Read the model definition and answer for the solid it produces. Units are mm, in the model's axes. Face numbers are marked on the shaded views. A direction names the side the tool comes from. Round coordinates to 2 decimals unless told otherwise and drop trailing zeros. Order: outer loops, then holes, each group sorted by start corner. A loop starts at its lowest first (then second) coordinate and runs counter-clockwise, first axis right, second up. Notation, with made-up numbers: (-30, 66) -> (5, 66) arc R6 cw to (5, 75) -> close; hole circle Ø2 at (-21, 16). An arc over 180 degrees is marked (long way). One line per item, written item: value. Start each with the question number.
1. Section B-B (z = 2.25) is taken. Give the vertices of the cut face in (x, y).
2. The mould has two halves that part along Y. Classify the marked faces 1, 2 and 3: released by +Y, released by -Y, zero draft, split by the parting line, or undercut.
3. Section A-A (x = 7.5) is taken. Give the vertices of the cut face in (y, z), then the cut area to 3 significant figures.
4. Section D-D (x = -3) is taken. Give the vertices of the cut face in (y, z).
5. Flat-ended cylindrical pins translate along their axes: pin 1 Ø10 at (x, z) = (-8, 5.5) entering from -Y; pin 2 Ø0.6 at (y, z) = (-16.5, 2.5) entering from -X. Find the tip coordinate at first contact, or state that the pin passes through.
6. Section C-C (y = -4.25) is taken. Give the vertices of the cut face in (x, z), then the cut area to 3 significant figures.
7. Consider line 1 (Y direction, x = 11, z = 3); line 2 (Y direction, x = -18, z = 4.5); line 3 (X direction, y = -15.5, z = 3.5). Determine where each line is inside the solid, lowest interval first.
8. For the marked faces 4, 5 and 6, determine the directions among +Z, -Z, +X, -X, +Y, -Y from which every point of the face is accessible in a straight line to the end or side of a thin tool.
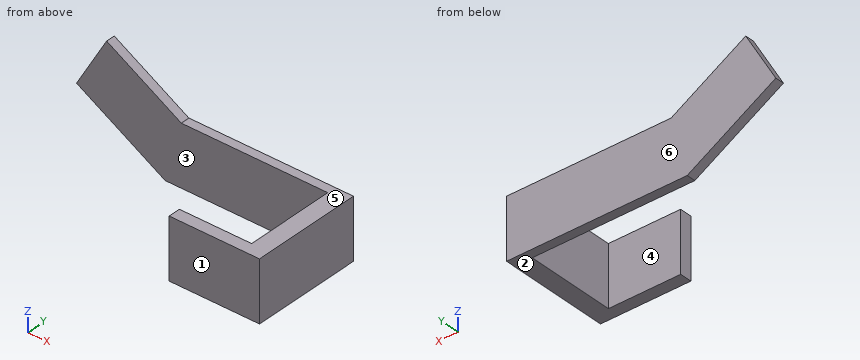
from build123d import *

# Parameters (mm, degrees)
BOSS_EXTRUDE1_DEPTH = 1.5
SKETCH2_W           = 3
SKETCH2_H           = 10
BOSS_EXTRUDE2_DEPTH = 17
SKETCH3_W           = 10
SKETCH3_H           = 2
BOSS_EXTRUDE3_DEPTH = 12


with BuildPart() as part:
    # Sketch1 → Boss-Extrude1 (new body)
    with BuildSketch(Plane(origin=(0, 0, 0), x_dir=(1, 0, 0), z_dir=(0, 1, 0))):
        Polygon((-10.606601718, 3.535533906), (-25.329033582, -4.964466094), (-20.329033582, -13.624720132), (-7.927109793, -6.464466094), (19.393398282, -6.464466094), (19.393398282, 3.535533906), align=None)
    extrude(amount=BOSS_EXTRUDE1_DEPTH)

    # Sketch2 → Boss-Extrude2 (add)
    with BuildSketch(Plane.XZ):
        with Locations((17.893398282, 1.464466094)):
            Rectangle(SKETCH2_W, SKETCH2_H)
    extrude(amount=BOSS_EXTRUDE2_DEPTH)

    # Sketch3 → Boss-Extrude3 (add)
    with BuildSketch(Plane.ZY.offset(-16.393398282)):
        with Locations((1.464466094, -16)):
            Rectangle(SKETCH3_W, SKETCH3_H)
    extrude(amount=BOSS_EXTRUDE3_DEPTH)


solid = part.part
Answer:
1. outline: (-20.63, 0) -> (16.39, 0) -> (16.39, -15) -> (4.39, -15) -> (4.39, -17) -> (19.39, -17) -> (19.39, 1.5) -> (-20.63, 1.5) -> close
2. face 1: released by -Y
2. face 2: zero draft
2. face 3: undercut
3. outline: (-17, -3.54) -> (-15, -3.54) -> (-15, 6.46) -> (-17, 6.46) -> close; (0, -3.54) -> (1.5, -3.54) -> (1.5, 6.46) -> (0, 6.46) -> close
3. area: 35.0 mm^2
4. outline: (0, -3.54) -> (1.5, -3.54) -> (1.5, 6.46) -> (0, 6.46) -> close
5. pin 1: y = 0
5. pin 2: x = 4.39
6. outline: (16.39, -3.54) -> (19.39, -3.54) -> (19.39, 6.46) -> (16.39, 6.46) -> close
6. area: 30.0 mm^2
7. line 1: -17 to -15, 0 to 1.5
7. line 2: 0 to 1.5
7. line 3: 4.39 to 19.39
8. face 4: +Z, -Z, -X
8. face 5: +Z, +X, +Y, -Y
8. face 6: +Z, -Z, +X, -X, +Y
